Check sheet for the drawn part. Datum: minimum x, y, z corner. Units: mm. A direction names the side the tool comes from. Round coordinates to 2 decimals unless told otherwise and drop trailing zeros. Order: outer loops, then holes, each group sorted by start corner. A loop starts at its lowest first (then second) coordinate and runs counter-clockwise, first axis right, second up.
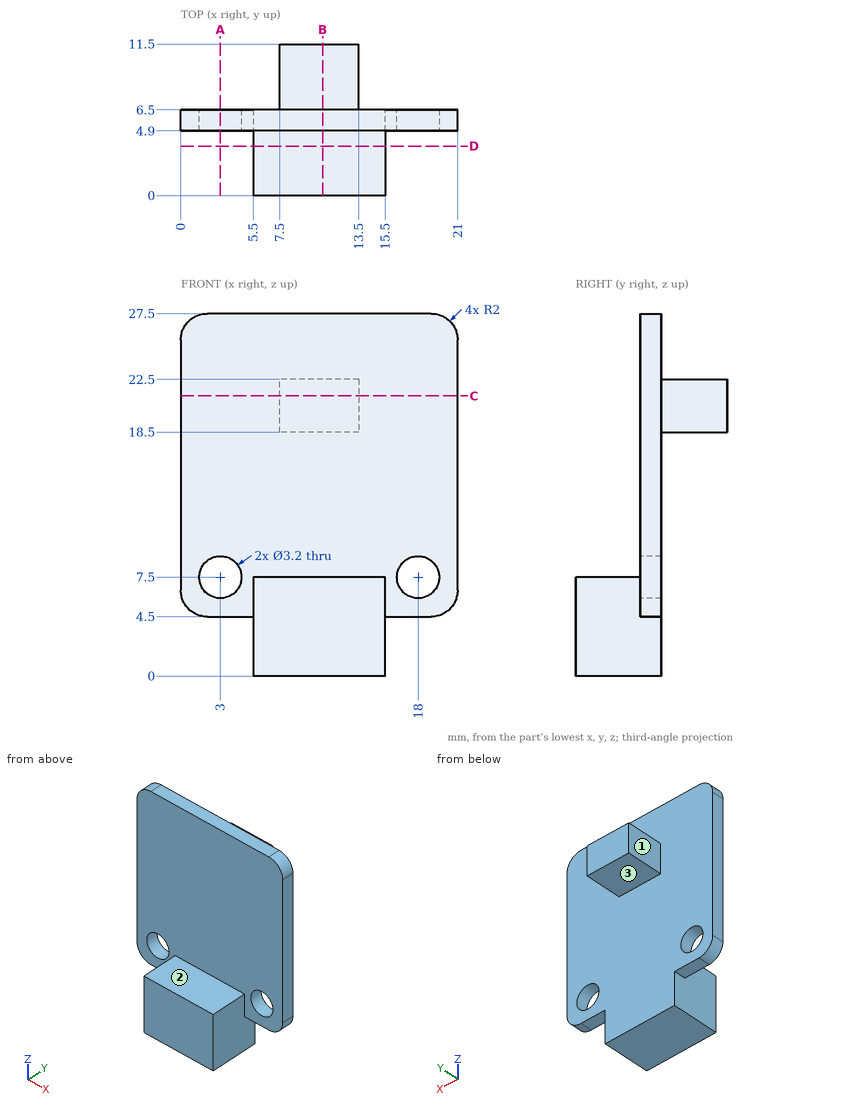
(1) Sectioned sample at A-A, the plane x = 3. Record the cut outline in (y, z), and give its area (3 significant figures).
Returned:
outline: (4.9, 4.5) - (6.5, 4.5) - (6.5, 5.9) - (4.9, 5.9) - close; (4.9, 9.1) - (6.5, 9.1) - (6.5, 27.5) - (4.9, 27.5) - close
area: 31.7 mm2
(2) Sectioned sample at D-D, the plane y = 3.75. Record the cut outline in (x, z), and give its area (3 significant figures).
Returned:
outline: (5.5, 0) - (15.5, 0) - (15.5, 7.5) - (5.5, 7.5) - close
area: 75.0 mm2
(3) Sectioned sample at B-B, the plane x = 10.75. Record the cut outline in (y, z), and give its area (3 significant figures).
Returned:
outline: (0, 0) - (6.5, 0) - (6.5, 18.5) - (11.5, 18.5) - (11.5, 22.5) - (6.5, 22.5) - (6.5, 27.5) - (4.9, 27.5) - (4.9, 7.5) - (0, 7.5) - close
area: 101 mm2
(4) Material ranges on line 1 (Z direction, x = 18, y = 5.65); line 2 (Z direction, x = 13, y = 9.75); line 3 (Z direction, x = 11, y = 2.5), recorded low to high.
Returned:
line 1: z = 4.5 to 5.9, 9.1 to 27.5
line 2: z = 18.5 to 22.5
line 3: z = 0 to 7.5
(5) Set-up check for the marked faces 1, 2 and 3: record each of +Z, -Z, +X, -X, +Y, -Y from which the full face is reachable in a straight line by a thin tool's end or side.
Returned:
face 1: +Z, -Z, -X, +Y
face 2: +Z, +X, -X, -Y
face 3: -Z, +X, -X, +Y
(6) Sectioned sample at C-C, the plane z = 21.25. Record the cut outline in (x, y), and give its area (3 significant figures).
Returned:
outline: (0, 4.9) - (21, 4.9) - (21, 6.5) - (13.5, 6.5) - (13.5, 11.5) - (7.5, 11.5) - (7.5, 6.5) - (0, 6.5) - close
area: 63.6 mm2
(7) Depth check by flat-ended pin: P1, Ø1.5, axis at x = 11, z = 23, coming from the -Y side; P2, Ø2, axis at y = 8, z = 21, coming from the +X side; P3, Ø5, axis at x = 18.5, y = 4, coming from the -Z side; P4, Ø12, axis at x = 11, z = 15.5, coming from the +Y side. Enter the tip coordinate at first touch or a pass-through.
Returned:
P1: stops at y = 4.9
P2: stops at x = 13.5
P3: stops at z = 4.5
P4: stops at y = 11.5
